```python
from build123d import *

# Parameters (mm, degrees)
BOSS_EXTRUDE1_DEPTH            = 33
M3X0_5_TAPPED_HOLE1_AT_2_COUNT = 2
M3X0_5_TAPPED_HOLE1_AT_2_PITCH = 43.840620434
M3X0_5_TAPPED_HOLE1_AT_3_COUNT = 2
M3X0_5_TAPPED_HOLE1_AT_3_PITCH = 31
M3X0_5_TAPPED_HOLE1_AT_4_COUNT = 2
M3X0_5_TAPPED_HOLE1_AT_4_PITCH = 31
SKETCH4_OUTSIDE_W              = 57.59
SKETCH4_OUTSIDE_H              = 57.59
CUT_EXTRUDE1_DEPTH             = 8
SKETCH5_W                      = 19
SKETCH5_H                      = 22
CUT_EXTRUDE2_DEPTH             = 1
CIRPATTERN1_COUNT              = 4
SKETCH7_R                      = 11
BOSS_EXTRUDE2_DEPTH            = 2
SKETCH8_R                      = 2.5
BOSS_EXTRUDE3_DEPTH            = 12.7
CUT_EXTRUDE3_DEPTH             = 7.2


with BuildPart() as part:
    # Sketch1 → Boss-Extrude1 (new body)
    with BuildSketch(Plane.XY):
        Polygon((16.757359313, 21), (-16.757359313, 21), (-21, 16.757359313), (-21, -16.757359313), (-16.757359313, -21), (16.757359313, -21), (21, -16.757359313), (21, 16.757359313), align=None)
    extrude(amount=-BOSS_EXTRUDE1_DEPTH)

    # Sketch2 → M3x0.5 Tapped Hole1 (revolve, cut)
    with BuildSketch(Plane(origin=(-15.5, 15.5, 0), x_dir=(0, -1, 0), z_dir=(1, 0, 0))):
        Polygon((0, 0), (0, 8.251075774), (1.25, 7.5), (1.25, 0), align=None)
    m3x0_5_tapped_hole1 = revolve(axis=Axis((-15.5, 15.5, 6.35), (0, 0, -1)), mode=Mode.SUBTRACT)

    # M3x0.5 Tapped Hole1 at 2: M3x0.5 Tapped Hole1 ×2
    with Locations(*[Vector(0.707106781, -0.707106781, 0) * (i * M3X0_5_TAPPED_HOLE1_AT_2_PITCH) for i in range(1, M3X0_5_TAPPED_HOLE1_AT_2_COUNT)]):
        add(m3x0_5_tapped_hole1, mode=Mode.SUBTRACT)

    # M3x0.5 Tapped Hole1 at 3: M3x0.5 Tapped Hole1 ×2
    with Locations(*[(i * M3X0_5_TAPPED_HOLE1_AT_3_PITCH, 0, 0) for i in range(1, M3X0_5_TAPPED_HOLE1_AT_3_COUNT)]):
        add(m3x0_5_tapped_hole1, mode=Mode.SUBTRACT)

    # M3x0.5 Tapped Hole1 at 4: M3x0.5 Tapped Hole1 ×2
    with Locations(*[(0, -i * M3X0_5_TAPPED_HOLE1_AT_4_PITCH, 0) for i in range(1, M3X0_5_TAPPED_HOLE1_AT_4_COUNT)]):
        add(m3x0_5_tapped_hole1, mode=Mode.SUBTRACT)

    # Sketch4 outside → Cut-Extrude1 (cut, symmetric)
    with BuildSketch(Plane.XY.offset(-16.5)):
        Rectangle(SKETCH4_OUTSIDE_W, SKETCH4_OUTSIDE_H)
        Polygon((11, -20), (-11, -20), (-20, -11), (-20, 11), (-11, 20), (11, 20), (20, 11), (20, -11), align=None, mode=Mode.SUBTRACT)
    extrude(amount=CUT_EXTRUDE1_DEPTH, both=True, mode=Mode.SUBTRACT)

    # Sketch5 → Cut-Extrude2 (cut)
    with BuildSketch(Plane(origin=(21, 0, 0), x_dir=(0, 0, -1), z_dir=(1, 0, 0))):
        with Locations((16.5, 0)):
            Rectangle(SKETCH5_W, SKETCH5_H)
    cut_extrude2 = extrude(amount=-CUT_EXTRUDE2_DEPTH, mode=Mode.SUBTRACT)

    # CirPattern1: Cut-Extrude2 ×4 about axis
    cirpattern1_axis = Axis((0, 0, 0), (0, 0, 1))
    for i in range(1, CIRPATTERN1_COUNT):
        add(cut_extrude2.rotate(cirpattern1_axis, i * 360 / CIRPATTERN1_COUNT), mode=Mode.SUBTRACT)

    # Sketch7 → Boss-Extrude2 (add)
    with BuildSketch(Plane.XY):
        Circle(SKETCH7_R)
    extrude(amount=BOSS_EXTRUDE2_DEPTH)

    # Sketch8 → Boss-Extrude3 (add)
    with BuildSketch(Plane.XY.offset(2)):
        Circle(SKETCH8_R)
    extrude(amount=BOSS_EXTRUDE3_DEPTH)

    # Sketch9 → Cut-Extrude3 (cut)
    with BuildSketch(Plane.XY.offset(14.7)):
        with BuildLine():
            Line((-1.5, 2), (1.5, 2))
            ThreePointArc((1.5, 2), (0, 2.5), (-1.5, 2))
        make_face()
    extrude(amount=-CUT_EXTRUDE3_DEPTH, mode=Mode.SUBTRACT)

    # Mirror1: M3x0.5 Tapped Hole1 across plane
    add(m3x0_5_tapped_hole1.mirror(Plane.XY.offset(-16.5)), mode=Mode.SUBTRACT)

    # Mirror1 copy 1 sketch → Mirror1 copy 1 (revolve, cut)
    with BuildSketch(Plane(origin=(15.5, -15.5, -33), x_dir=(0, -1, 0), z_dir=(1, 0, 0))):
        Polygon((0, 0), (0, -8.251075774), (1.25, -7.5), (1.25, 0), align=None)
    revolve(axis=Axis((15.5, -15.5, -39.35), (0, 0, -1)), mode=Mode.SUBTRACT)

    # Mirror1 copy 2 sketch → Mirror1 copy 2 (revolve, cut)
    with BuildSketch(Plane(origin=(15.5, 15.5, -33), x_dir=(0, -1, 0), z_dir=(1, 0, 0))):
        Polygon((0, 0), (0, -8.251075774), (1.25, -7.5), (1.25, 0), align=None)
    revolve(axis=Axis((15.5, 15.5, -39.35), (0, 0, -1)), mode=Mode.SUBTRACT)

    # Mirror1 copy 3 sketch → Mirror1 copy 3 (revolve, cut)
    with BuildSketch(Plane(origin=(-15.5, -15.5, -33), x_dir=(0, -1, 0), z_dir=(1, 0, 0))):
        Polygon((0, 0), (0, -8.251075774), (1.25, -7.5), (1.25, 0), align=None)
    revolve(axis=Axis((-15.5, -15.5, -39.35), (0, 0, -1)), mode=Mode.SUBTRACT)


solid = part.part
```
Design review of the part built by this model. Coordinates are the model's own, in mm. A direction names the side the tool comes from. Give positions to 0.01 mm unless a question says otherwise; leave off trailing zeros. Loops run counter-clockwise (first coordinate to the right, second up) from the corner with the lowest first, then second, coordinate; pieces in that order, holes last. Notation, with made-up numbers: (76.5, 57.25) -> (88.5, 57.25) arc R16 cw to (88.5, 88.25) -> close; hole circle Ø4 at (-16, 32.5). An arc over 180 degrees is marked (long way). One line per item, written item: value.
Q1. We need section B-B on z = -14.5. Give the boundary of the cut face in (x, y), and give its area (3 significant figures).
Numbers:
outline: (-20, -11) -> (-11, -20) -> (11, -20) -> (20, -11) -> (20, 11) -> (11, 20) -> (-11, 20) -> (-20, 11) -> close
area: 1,440 mm^2
Q2. Draft analysis for pull direction Y (two halves, no side actions). For faces 1 (the flat face through (0, -20, -16)), 2 (the flat face through (0, 0, 14.7)), 3 (the cylindrical face through (14.26, -15.34, -29.3)), 4 (the flat face through (0, 2, 11)), state which applies: pulls with the +Y half, pulls with the -Y half, needs draft (parallel to the pull), parting line crosses it, or undercut.
Numbers:
face 1: pulls with the -Y half
face 2: needs draft
face 3: undercut
face 4: pulls with the +Y half
Q3. For pin 1 Ø3 at (x, y) = (10, -15) entering from +Z; pin 2 Ø5 at (y, z) = (-13, -14.5) entering from -X; pin 3 Ø0.8 at (y, z) = (20.5, -25.5) entering from -X; pin 4 Ø1.5 at (y, z) = (-4, 9.5) entering from +X, all flat-tipped, find the tip position at first contact; note any pin that passes through.
Numbers:
pin 1: stops at z = 0
pin 2: stops at x = -20
pin 3: stops at x = -17.66
pin 4: passes through
Q4. Machinability: for faces 5 (the flat face through (20, 0, -16)), 6 (the flat face through (-18.91, -18.85, -4.19)), 7 (the cylindrical face through (-2.38, -10.74, 0.99)), 8 (the cylindrical face through (-16.345, -14.579, -29.303)), 9 (the flat face through (17, 17, -8.5)), which of the approach directions +Z, -Z, +X, -X, +Y, -Y give a long, thin tool a straight path to every point of the face, cutting with its end or side? Answer none if there is none.
Numbers:
face 5: +X
face 6: +Z, -Z, -X, -Y
face 7: +Z
face 8: -Z
face 9: +X, +Y
Q5. We need section A-A on y = -12.5. Give the boundary of the cut face in (x, z), and give its area (3 significant figures).
Numbers:
outline: (-21, -33) -> (21, -33) -> (21, -24.5) -> (18.5, -24.5) -> (18.5, -8.5) -> (21, -8.5) -> (21, 0) -> (-21, 0) -> (-21, -8.5) -> (-18.5, -8.5) -> (-18.5, -24.5) -> (-21, -24.5) -> close
area: 1,310 mm^2
Q6. We need section C-C on x = 0.5. Give the boundary of the cut face in (y, z).
Numbers:
outline: (-21, -33) -> (21, -33) -> (21, -26) -> (20, -26) -> (20, -7) -> (21, -7) -> (21, 0) -> (10.99, 0) -> (10.99, 2) -> (2.45, 2) -> (2.45, 7.5) -> (2, 7.5) -> (2, 14.7) -> (-2.45, 14.7) -> (-2.45, 2) -> (-10.99, 2) -> (-10.99, 0) -> (-21, 0) -> (-21, -7) -> (-20, -7) -> (-20, -26) -> (-21, -26) -> close
Q7. We need section D-D on z = 4. Give the boundary of the cut face in (x, y), and give its area (3 significant figures).
Numbers:
outline: circle Ø5 at (0, 0)
area: 19.6 mm^2
Q8. For L1, parallel to X at y = 15.5, z = -26.75; L2, parallel to X at y = 15, z = -1, list the stretches that pass through material, from the lowest coordinate up.
Numbers:
L1: x = -21 to -16.75, -14.25 to 14.25, 16.75 to 21
L2: x = -21 to -16.65, -14.35 to 14.35, 16.65 to 21
